Verification items for this drawing (mm, ordinates from the low corner). Round coordinates to 2 decimals unless told otherwise and drop trailing zeros. Order: outer loops, then holes, each group sorted by start corner. A loop starts at its lowest first (then second) coordinate and runs counter-clockwise, first axis right, second up. Notation, with made-up numbers: (-13, -26.5) -> (41, -26.5) arc R20 ccw to (41, -5.5) -> close; hole circle Ø5 at (-10.5, 39.5). An arc over 180 degrees is marked (long way). Answer in a Markdown table with one row per item. Add a question column.
1. Material ranges on L1, parallel to X at y = 12.5, z = 5.5; L2, parallel to X at y = 6.25, z = 8 (1 decimal); L3, parallel to Y at x = 25.4, z = 6.5, recorded low to high. Write a range as from..to.
2. Sectioned sample at B-B, the plane z = 8. Record the boundary of the cut face in (x, y) (1 decimal), then the cut area to 3 significant figures.
3. Sectioned sample at C-C, the plane y = 12.7. Count the separate pieces of the cut face and the enclosed holes in it, then the cut area to 3 significant figures.
4. Sectioned sample at D-D, the plane z = 13. Record the boundary of the cut face in (x, y) (1 decimal), then the cut area to 3 significant figures.
5. Sectioned sample at A-A, the plane x = 38.1. Record the boundary of the cut face in (y, z), then the cut area to 3 significant figures.
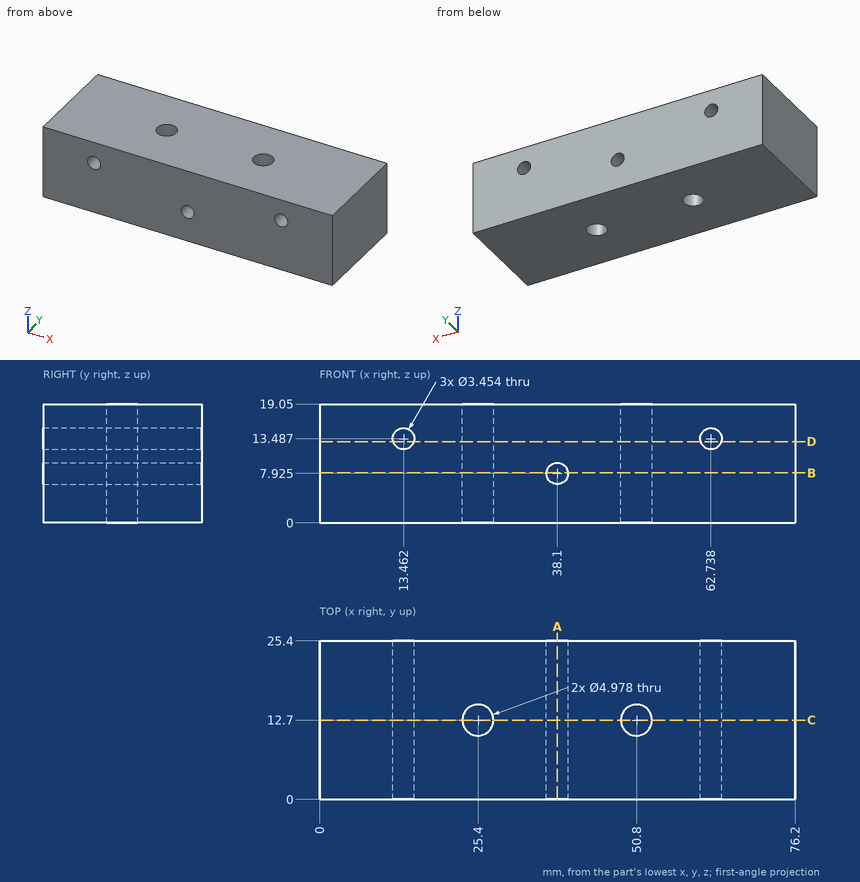
Answer key:
| question | item | result |
|---|---|---|
| 1 | L1 | x = 0..22.92, 27.88..48.32, 53.28..76.2 |
| 1 | L2 | x = 0..36.4, 39.8..76.2 |
| 1 | L3 | y = 0..10.21, 15.19..25.4 |
| 2 | outline | (0, 0) -> (36.4, 0) -> (36.4, 25.4) -> (0, 25.4) -> close; (39.8, 0) -> (76.2, 0) -> (76.2, 25.4) -> (39.8, 25.4) -> close; hole circle Ø5 at (25.4, 12.7); hole circle Ø5 at (50.8, 12.7) |
| 2 | area | 1,810 mm² |
| 3 | separate pieces | 3 |
| 3 | enclosed holes | 3 |
| 3 | area | 1,230 mm² |
| 4 | outline | (0, 0) -> (11.8, 0) -> (11.8, 25.4) -> (0, 25.4) -> close; (15.1, 0) -> (61.1, 0) -> (61.1, 25.4) -> (15.1, 25.4) -> close; (64.4, 0) -> (76.2, 0) -> (76.2, 25.4) -> (64.4, 25.4) -> close; hole circle Ø5 at (25.4, 12.7); hole circle Ø5 at (50.8, 12.7) |
| 4 | area | 1,730 mm² |
| 5 | outline | (0, 0) -> (25.4, 0) -> (25.4, 6.2) -> (0, 6.2) -> close; (0, 9.65) -> (25.4, 9.65) -> (25.4, 19.05) -> (0, 19.05) -> close |
| 5 | area | 396 mm² |
